Source: CAD feature listing. Evaluate the final solid. Frame: model axes, mm. A direction names the side the tool comes from. Coordinates: 2 decimals unless noted, no trailing zeros. Write each loop counter-clockwise with the first axis right and the second up, starting at its lowest first coordinate (ties: lowest second). Pieces come first, ordered by that corner, then holes. Notation, with made-up numbers: (78, 84.25) -> (119, 84.25) arc R16 ccw to (119, 100.25) -> close; hole circle Ø11 at (72, -32). An arc over 180 degrees is marked (long way). Write item = value, one per line.
Autodesk Inventor part; units mm, degrees
ref_plane "YZ Plane" through (0, 0, 0) normal (1, 0, 0) x (0, 1, 0)
ref_plane "XZ Plane" through (0, 0, 0) normal (0, 1, 0) x (-1, 0, 0)
ref_plane "XY Plane" through (0, 0, 0) normal (0, 0, 1) x (1, 0, 0)
sketch "Sketch1" plane through (0, 0, 0) normal (0, 1, 0) x (-1, 0, 0)
  circle A0 centre (0, 0) radius 72.39
  circle A1 centre (0, 0) radius 69.85
  arc A2 (-76.197, 3.807) -> (-76.197, -3.807) centre (-76.197, 0) ccw
  circle A3 centre (-76.197, 0) radius 2.286
  line L0 (-76.197, 3.807) -> (-72.2898, 3.807)
  line L1 (-76.197, -3.807) -> (-72.2898, -3.807)
  dimension "d0" = 144.78
  dimension "d1" = 139.7
  dimension "d2" = 4.572
extrude "Extrusion1" add sketch "Sketch1" along normal blind 50.8
sketch "Sketch2" plane through (0, 50.8, 0) normal (0, 1, 0) x (1, 0, 0)
  circle A0 centre (76.197, 0) radius 2.286
  circle A1 centre (0, 0) radius 76.197
  arc A2 (-76.1019, 3.8058) -> (-76.1019, -3.8058) centre (-76.197, 0) ccw
  arc A3 (72.2898, 3.807) -> (72.2898, -3.807) centre (0, 0) ccw
  arc A4 (-76.1627, 2.2857) -> (-76.1627, -2.2857) centre (-76.197, 0) ccw
  line L0 (-76.197, -3.807) -> (-72.2898, -3.807)
  line L1 (-76.197, 3.807) -> (-72.39, 3.807)
  line L2 (-51.1875, 51.1875) -> (-53.8794, 53.8794)
  line L3 (0, 0) -> (76.197, 0) construction
  line L4 (0, 0) -> (76.197, 0) construction
  arc A5 (-56.5033, -51.1211) -> (-50.7603, -56.0621) centre (-53.8794, -53.8794) ccw
  line L5 (-51.1211, -56.5033) -> (-48.7078, -53.5524)
  line L6 (-56.5033, -51.1211) -> (-53.744, -48.4963)
  circle A6 centre (-53.8794, -53.8794) radius 2.286
  circle A7 centre (-53.8794, 53.8794) radius 2.286
  line L7 (-57.0474, 50.5132) -> (-54.2736, 47.9029)
  line L8 (-50.5132, 57.0474) -> (-47.9029, 54.2736)
  arc A8 (-50.5132, 57.0474) -> (-57.0474, 50.5132) centre (-53.8794, 53.8794) ccw
  line L9 (0, 0) -> (-26.9652, -26.9652)
  circle A9 centre (-76.197, 0) radius 2.286
  point P0 (-76.1627, -2.2857)
  dimension "d5" = 4.572
  dimension "d6" = 135
  dimension "d8" = 4.572
  dimension "d9" = 4.572
extrude "Extrusion2" add sketch "Sketch2" against normal blind 25.4 contours L8 A3 L2 A7 A1 | A1 A7 A8 | A5 A1 A6 | A1 A6 L6 A3 L5 | L7 A3 L0 A1 A9 | A1 A7 L2 A3 L7 | A1 L0 A3 L6 | A1 A4 A2
sketch "Sketch3" plane through (0, 0, 0) normal (0, -1, 0) x (1, 0, 0)
  line L0 (72.2898, 3.807) -> (76.197, 3.807)
  circle A0 centre (0, 0) radius 72.39
  circle A1 centre (0, 0) radius 69.85
  line L1 (-69.85, 0) -> (52.6357, 45.9184)
  circle A2 centre (0, 0) radius 69.85
  line L2 (-69.85, 0) -> (52.6357, -45.9184)
  line L3 (52.6357, 45.9184) -> (55.1695, 46.8683)
  arc A3 (72.2898, 3.807) -> (-48.7078, 53.5524) centre (0, 0) ccw
  line L4 (52.6357, -45.9184) -> (55.1695, -46.8683)
  dimension "d12" = 130.81
extrude "Extrusion3" add sketch "Sketch3" along normal blind 19.05 contours A0 L4 A1 L3 picked at (58.6234, 40.6965)
sketch "Sketch4" plane through (0, 0, 0) normal (0, -1, 0) x (1, 0, 0)
  circle A0 centre (76.197, 0) radius 2.286
  circle A1 centre (76.197, 0) radius 2.286
  arc A2 (76.197, -3.807) -> (76.197, 3.807) centre (76.197, 0) ccw
  line L0 (76.197, -3.807) -> (72.2898, -3.807)
  line L1 (76.197, -3.807) -> (72.2898, -3.807)
  line L2 (72.2898, 3.807) -> (76.197, 3.807)
  line L3 (76.197, 3.807) -> (72.2898, 3.807)
  arc A3 (72.2898, -3.807) -> (72.2898, 3.807) centre (0, 0) ccw
  line L4 (72.2898, 3.807) -> (72.2898, -3.807)
  circle A4 centre (0, 0) radius 76.197
  line L5 (0, 0) -> (76.197, 0) construction
  line L6 (0, 0) -> (76.197, 0) construction
  arc A5 (67.8091, 34.755) -> (64.0033, 41.3469) centre (65.9886, 38.0985) ccw
  arc A6 (64.0033, -41.3469) -> (67.8091, -34.755) centre (65.9886, -38.0985) ccw
  circle A7 centre (65.9886, -38.0985) radius 2.286
  circle A8 centre (65.9886, 38.0985) radius 2.286
  line L7 (64.0033, 41.3469) -> (60.7024, 39.4402)
  line L8 (67.8091, 34.755) -> (64.4936, 32.8768)
  arc A9 (55.1695, -46.8683) -> (55.1695, 46.8683) centre (0, 0) ccw
  line L9 (67.8105, -34.7524) -> (64.4936, -32.8768)
  line L10 (64.0017, -41.3494) -> (60.6368, -39.541)
  line L11 (64.0088, 36.9555) -> (65.9886, 38.0985)
  line L12 (62.689, -36.1935) -> (62.6916, -36.195)
  line L13 (64.0088, -36.9555) -> (65.9886, -38.0985)
  arc A10 (62.7648, -36.068) -> (62.6181, -36.3219) centre (65.9886, -38.0985) ccw
  arc A11 (64.0017, -41.3494) -> (67.8105, -34.7524) centre (65.9886, -38.0985) ccw
  point P0 (76.1019, -3.807)
  point P1 (76.1019, 3.807)
  dimension "d18" = 4.572
  dimension "d19" = 4.572
extrude "Extrusion4" add sketch "Sketch4" along normal blind 19.05 contours A0 A4 L2 A2 L0 | A0 A4 L0 A3 L2 | L2 A9 L8 A4 | A4 L9 A9 L0 | L8 A9 L7 A4 A8 | A4 A8 A5 | A11 A4 A6 | A4 A7 L10 A9 L9 | A6 A4 A7
sketch "Sketch5" plane through (0, 25.4, 0) normal (0, -1, 0) x (1, 0, 0)
  circle A0 centre (-76.197, 0) radius 2.286
  circle A1 centre (-76.197, 0) radius 2.286
  arc A2 (-76.1019, 3.8058) -> (-76.1019, -3.8058) centre (-76.197, 0) ccw
  arc A3 (-76.1019, -3.8058) -> (-57.0474, -50.5132) centre (0, 0) ccw
  line L0 (-76.1019, -3.8058) -> (-72.2948, -3.7107)
  arc A4 (-48.7078, 53.5524) -> (-47.9029, -54.2736) centre (0, 0) ccw
  arc A5 (-56.5033, 51.1211) -> (-76.1019, 3.8058) centre (0, 0) ccw
  line L1 (-76.1019, 3.8058) -> (-72.2948, 3.8058)
  line L2 (-72.2948, -3.7107) -> (-72.2948, 3.8058)
  point P0 (-72.2948, 3.7107)
extrude "Extrusion5" add sketch "Sketch5" along normal blind 44.45 contours L1 L2 A4 L0 A2
properties part number "NewShooterCup"
1) Cut plane C-C, the plane z = 17. Output: boundary loops of the cut face in (x, y), and give its area (3 significant figures).
Answer block:
outline = (-74.28, 25.4) -> (-70.37, 25.4) -> (-70.37, 0) -> (-67.75, 0) -> (-67.75, 50.8) -> (-74.28, 50.8) -> close; (67.75, -19.05) -> (74.28, -19.05) -> (74.28, 0) -> (70.37, 0) -> (70.37, 50.8) -> (67.75, 50.8) -> close
area = 489 mm2
2) First-contact query: pin 1 Ø3 at (x, y) = (75, 10.5) entering from -Z; pin 2 Ø1.5 at (y, z) = (23, 8) entering from -X; pin 3 Ø2.5 at (x, z) = (76.197, 0) entering from +Y; pin 4 Ø7.5 at (x, z) = (65.99, 38.1) entering from +Y. Flat tips, straight axial feed; report the tip coordinate or a pass-through.
Answer block:
pin_1 = -3.81
pin_2 = -72.03
pin_3 = through
pin_4 = 0
3) Cut plane A-A, the plane y = -6.5. Give the number of separate pieces and of enclosed holes in the cut face, and give its area (3 significant figures).
Answer block:
separate_pieces = 2
enclosed_holes = 4
area = 637 mm2
4) Pull-direction query (X, two-part tool) for faces 5 (the cylindrical face through (-55.56, 38.28, 52.33)), 6 (the cylindrical face through (73.54, -9.39, 19.94)), 7 (the cylindrical face through (-56.63, 38.28, 56.51)), 8 (the flat face through (70, -19.05, 0)); classes: +X half, -X half, draft (parallel to the pull), parting line (faces both ways), or undercut.
Answer block:
face_5 = undercut
face_6 = +X half
face_7 = undercut
face_8 = draft
5) Cut plane B-B, the plane x = 0. Output: boundary loops of the cut face in (y, z).
Answer block:
outline = (0, -72.39) -> (50.8, -72.39) -> (50.8, -69.85) -> (0, -69.85) -> close; (0, 69.85) -> (50.8, 69.85) -> (50.8, 72.39) -> (0, 72.39) -> close
6) Material intervals for probe 1 along Z at (x, y) = (1, 41); probe 2 along X at (y, z) = (26.5, -1.5); probe 3 along X at (y, z) = (12, 43), sorted ascending. Write a range as [from, to].
Answer block:
probe_1 = [-72.38, -69.84], [69.84, 72.38]
probe_2 = [-79.7, -77.92], [-74.47, -69.83], [69.83, 74.47], [77.92, 79.7]
probe_3 = [-58.23, -55.05], [55.05, 58.23]
7) Reachability of faces 1 (the flat face through (-74, -19.05, -2)), 2 (the cylindrical face through (1.491, 24.125, -72.375)), 3 (the cylindrical face through (-72.39, -9.39, -0.05)), 4 (the flat face through (-74, 3, 3.806)) from +Z, -Z, +X, -X, +Y, -Y: full face, straight path, thin tool, end or side. Return the list, or none.
Answer block:
face_1 = +Z, -Z, +X, -X, -Y
face_2 = -Z
face_3 = -Y
face_4 = +Z, -X, -Y
